For this review, use the dimensioned drawing (mm, ordinates from the lowest corner) and the shaded views. Round coordinates to 2 decimals unless told otherwise and drop trailing zeros. Order: outer loops, then holes, each group sorted by start corner. A loop starts at its lowest first (then second) coordinate and runs counter-clockwise, first axis right, second up. Notation, with made-up numbers: (18.5, 83) - (75.5, 83) arc R25 ccw to (75.5, 116) - close; hole circle Ø3 at (33.5, -34). An arc over 180 degrees is marked (long way). Write each question's results on one line, items separated by ' | '. Start each with the question number.
(1) Take a section at C-C, the plane x = 95. Give the boundary of the cut face in (y, z).
(2) Take a section at A-A, the plane y = 4. Give the boundary of the cut face in (x, z).
(3) For L1, parallel to Z at x = 7, y = 6.25; L2, parallel to X at y = 4.75, z = 4; L3, parallel to X at y = 4.5, z = 3.5, list the stretches that pass through material, from the lowest coordinate up. Write a range as from..to.
(4) Take a section at B-B, the plane z = 4. Give the boundary of the cut face in (x, y).
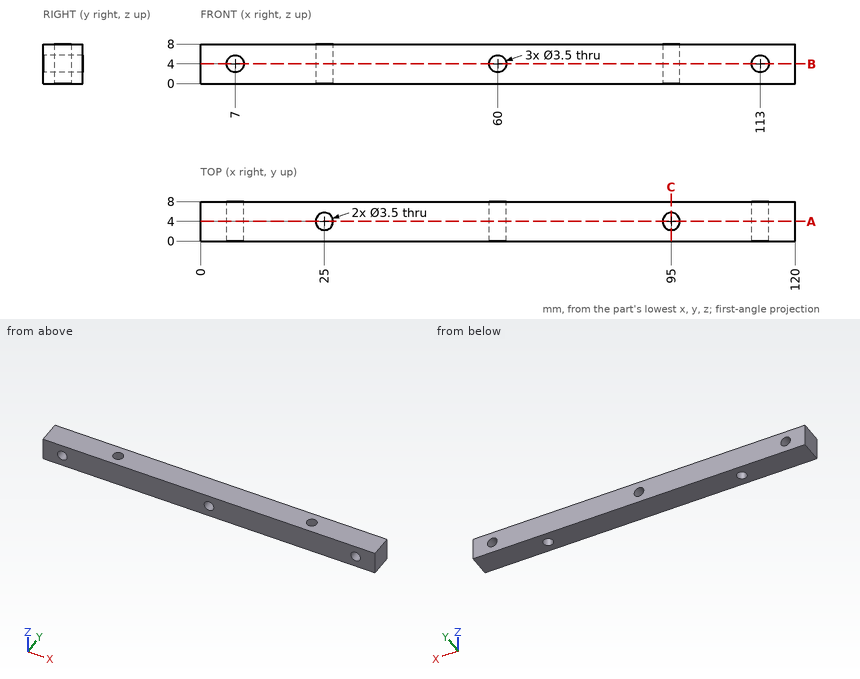
Results below:
1) outline: (0, 0) - (2.25, 0) - (2.25, 8) - (0, 8) - close; (5.75, 0) - (8, 0) - (8, 8) - (5.75, 8) - close
2) outline: (0, 0) - (23.25, 0) - (23.25, 8) - (0, 8) - close; (26.75, 0) - (93.25, 0) - (93.25, 8) - (26.75, 8) - close; (96.75, 0) - (120, 0) - (120, 8) - (96.75, 8) - close; hole circle Ø3.5 at (7, 4); hole circle Ø3.5 at (60, 4); hole circle Ø3.5 at (113, 4)
3) L1: z = 0..2.25, 5.75..8 | L2: x = 0..5.25, 8.75..23.42, 26.58..58.25, 61.75..93.42, 96.58..111.25, 114.75..120 | L3: x = 0..5.32, 8.68..23.32, 26.68..58.32, 61.68..93.32, 96.68..111.32, 114.68..120
4) outline: (0, 0) - (5.25, 0) - (5.25, 8) - (0, 8) - close; (8.75, 0) - (58.25, 0) - (58.25, 8) - (8.75, 8) - close; (61.75, 0) - (111.25, 0) - (111.25, 8) - (61.75, 8) - close; (114.75, 0) - (120, 0) - (120, 8) - (114.75, 8) - close; hole circle Ø3.5 at (25, 4); hole circle Ø3.5 at (95, 4)
